```python
from build123d import *

# Parameters (mm, degrees)
CUT_EXTRUDE_START        = 5
SKETCH_2_R               = 8
CUT_EXTRUDE_1_DEPTH      = 8
CUT_EXTRUDE_2_DEPTH      = 21.420577857
CUT_EXTRUDE_2_DEPTH_BACK = 21.420577857
SKETCH_3_R               = 6


with BuildPart() as part:
    # 草图1 → 旋转1 (revolve)
    with BuildSketch(Plane.XY, mode=Mode.PRIVATE) as revolve_1_sk:
        Polygon((0, 5), (10, 5), (14, 3.2), (14, -3.2), (10, -5), (0, -5), align=None)
    revolve(revolve_1_sk.sketch.rotate(Axis((0, -5, 0), (0, 1, 0)), 90), axis=Axis((0, -5, 0), (0, 1, 0)))

    # 草图2 → 切除-拉伸1 (cut)
    with BuildSketch(Plane(origin=(0, 0, 0), x_dir=(1, 0, 0), z_dir=(0, 1, 0)).offset(CUT_EXTRUDE_START)):
        with Locations(Location((0, 0, 0), (0, 0, 270))):
            Circle(SKETCH_2_R)
    extrude(amount=-CUT_EXTRUDE_1_DEPTH, mode=Mode.SUBTRACT)

    # 草图3 → 切除-拉伸2 (cut, two sides: drawn at the far end of the back side and taken through both)
    with BuildSketch(Plane(origin=(0, 0, 0), x_dir=(1, 0, 0), z_dir=(0, 1, 0)).offset(-CUT_EXTRUDE_2_DEPTH_BACK)):
        with Locations(Location((0, 0, 0), (0, 0, 270))):
            Circle(SKETCH_3_R)
    extrude(amount=CUT_EXTRUDE_2_DEPTH + CUT_EXTRUDE_2_DEPTH_BACK, mode=Mode.SUBTRACT)


solid = part.part
```
Input: part model. Units: mm. Frame: model coordinates. A direction names the side the tool comes from. Coordinates: 2 decimals unless noted, no trailing zeros. Write each loop counter-clockwise with the first axis right and the second up, starting at its lowest first coordinate (ties: lowest second). Pieces come first, ordered by that corner, then holes. Notation, with made-up numbers: (29, -35) - (74, -35) arc R16 cw to (74, -24) - close; hole circle Ø8 at (68.25, 22.25). An arc over 180 degrees is marked (long way). Put each result on its own line as item: value. Start each with the question number.
1) Cut plane A-A (z = 0). Return the cut outline in (x, y).
2) Mould query, pull axis X, two halves, no side actions, for faces 3 (the face through (1.802, -4.014, 5.723)), 4 (the face through (-8.2, 5, 0)), 5 (the face through (12.4, 0, -6.5)). Classes: pulls with the +X half, pulls with the -X half, needs draft (parallel to the pull), parting line crosses it, or undercut.
3) Cut plane C-C (y = -3.75). Return the cut outline in (x, z), plus the area to 3 significant figures.
4) Ray query, L1, parallel to X at y = 2.5, z = 0; L2, parallel to X at y = -4.05, z = 0; L3, parallel to Z at x = -7.25, y = 0.25. Return the intervals inside material, ascending.
5) Contact query for flat-ended pins moving along their axis: pin 1 (15.5 mm diameter, centred on x = 0, z = 0, fed in from +Y); pin 2 (1 mm diameter, centred on x = 6.5, z = -8.5, fed in from +Y); pin 3 (1.5 mm diameter, centred on x = 7.5, y = 2.5, fed in from +Z); pin 4 (12 mm diameter, centred on x = -8, z = -11, fed in from +Y). Output: stop coordinate, or through.
6) Cut plane D-D (y = 2.5). Return the cut outline in (x, z), plus the area to 3 significant figures.
7) Reachability of faces 1 (the face through (6, -3, -2)), 2 (the face through (-3.062, -4.913, -9.723)) from +Z, -Z, +X, -X, +Y, -Y: full face, straight path, thin tool, end or side. Return the list, or none.
8) Cut plane B-B (x = 0). Return the cut outline in (y, z), plus the area to 3 significant figures.
Resolved:
1. outline: (-14, -3.2) - (-10, -5) - (-6, -5) - (-6, -3) - (-8, -3) - (-8, 5) - (-10, 5) - (-14, 3.2) - close; (6, -5) - (10, -5) - (14, -3.2) - (14, 3.2) - (10, 5) - (8, 5) - (8, -3) - (6, -3) - close
2. face 3: undercut
2. face 4: needs draft
2. face 5: parting line crosses it
3. outline: circle Ø25.56 at (0, 0); hole circle Ø12 at (0, 0)
3. area: 400 mm2
4. L1: x = -14 to -8, 8 to 14
4. L2: x = -12.11 to -6, 6 to 12.11
4. L3: z = -11.98 to -3.38, 3.38 to 11.98
5. pin 1: stops at y = -3
5. pin 2: stops at y = 4.91
5. pin 3: stops at z = 12.27
5. pin 4: stops at y = 5
6. outline: circle Ø28 at (0, 0); hole circle Ø16 at (0, 0)
6. area: 415 mm2
7. face 1: +Y
7. face 2: -Y
8. outline: (-5, -10) - (-3.2, -14) - (3.2, -14) - (5, -10) - (5, -8) - (-3, -8) - (-3, -6) - (-5, -6) - close; (-5, 6) - (-3, 6) - (-3, 8) - (5, 8) - (5, 10) - (3.2, 14) - (-3.2, 14) - (-5, 10) - close
8. area: 114 mm2
